Read the model definition and answer for the solid it produces. Units are mm, in the model's axes. Coordinates: 2 decimals unless noted, no trailing zeros. Write each loop counter-clockwise with the first axis right and the second up, starting at its lowest first coordinate (ties: lowest second). Pieces come first, ordered by that corner, then holes. Notation, with made-up numbers: (38, 64) -> (82, 64) arc R28 ccw to (82, 100) -> close; hole circle Ø10 at (-0.5, 86). An arc over 180 degrees is marked (long way). One line per item, written item: value. Start each with the question number.
1. Find section B-B, the plane z = 3.75. Write down the section's boundary in (x, y).
2. Find section D-D, the plane x = 14.5. Write down the section's boundary in (y, z).
3. Consider line 1 along X through (y, z) = (0.5, 4); line 2 along Y through (x, z) = (61.5, 5.75); line 3 along X through (y, z) = (-51, 6). Determine where each line is inside the solid, lowest interval first.
4. Given P1, Ø8, axis at x = 0, y = -62.5, coming from the -Z side; P2, Ø1.5, axis at x = 12.5, z = 7, coming from the -Y side, each flat-ended and moving along its own axis, determine where each tip first touches the part or whether it passes through.
5. Find section A-A, the plane y = 0. Write down the section's boundary in (x, z).
6. Find section C-C, the plane x = 62.5. Write down the section's boundary in (y, z).
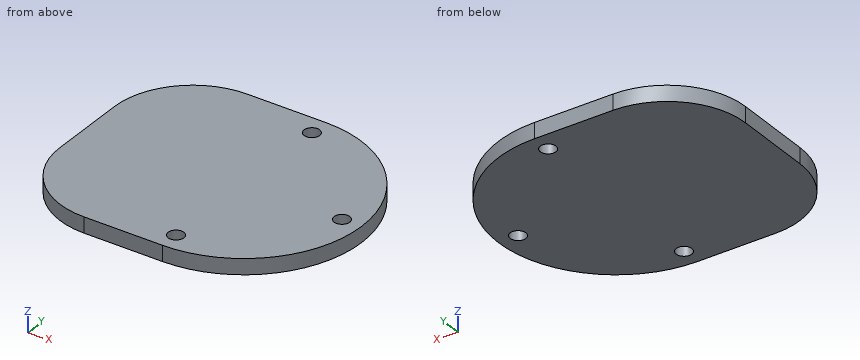
```python
from build123d import *

# Parameters (mm, degrees)
BOSS_EXTRUDE1_DEPTH = 10
SKETCH2_R           = 5
CUT_EXTRUDE1_DEPTH  = 10
FILLET1_R           = 50


with BuildPart() as part:
    # Sketch1 → Boss-Extrude1 (new body)
    with BuildSketch(Plane.XY):
        with BuildLine():
            Line((0, 75), (-100, 75))
            Line((-100, 75), (-100, -75))
            Line((-100, -75), (0, -75))
            ThreePointArc((0, -75), (75, 0), (0, 75))
        make_face()
    extrude(amount=BOSS_EXTRUDE1_DEPTH)

    # Sketch2 → Cut-Extrude1 (cut)
    with BuildSketch(Plane.XY.offset(10)):
        with Locations((0, 62.5)):
            Circle(SKETCH2_R)
        with Locations((62.5, 0)):
            Circle(SKETCH2_R)
        with Locations((0, -62.5)):
            Circle(SKETCH2_R)
    extrude(amount=-CUT_EXTRUDE1_DEPTH, mode=Mode.SUBTRACT)

    # Fillet1
    fillet1_edges = [part.edges().sort_by_distance(p)[0] for p in [
        (-100, -75, 5),
        (-100, 75, 5),
    ]]
    fillet(fillet1_edges, radius=FILLET1_R)


solid = part.part
```
Answer block:
1. outline: (-100, -25) arc R50 ccw to (-50, -75) -> (0, -75) arc R75 ccw to (0, 75) -> (-50, 75) arc R50 ccw to (-100, 25) -> close; hole circle Ø10 at (0, -62.5); hole circle Ø10 at (0, 62.5); hole circle Ø10 at (62.5, 0)
2. outline: (-73.58, 0) -> (73.58, 0) -> (73.58, 10) -> (-73.58, 10) -> close
3. line 1: x = -100 to 57.53, 67.47 to 75
3. line 2: y = -42.93 to -4.9, 4.9 to 42.93
3. line 3: x = -92.71 to 54.99
4. P1: passes through
4. P2: stops at y = -74.07
5. outline: (-100, 0) -> (57.5, 0) -> (57.5, 10) -> (-100, 10) -> close; (67.5, 0) -> (75, 0) -> (75, 10) -> (67.5, 10) -> close
6. outline: (-41.46, 0) -> (-5, 0) -> (-5, 10) -> (-41.46, 10) -> close; (5, 0) -> (41.46, 0) -> (41.46, 10) -> (5, 10) -> close
